Geometry check sheet. Reference: the model listing, model coordinates, mm. Face numbers are marked on the shaded views. A direction names the side the tool comes from. Round coordinates to 2 decimals unless told otherwise and drop trailing zeros. Write each loop counter-clockwise with the first axis right and the second up, starting at its lowest first coordinate (ties: lowest second). Pieces come first, ordered by that corner, then holes. Notation, with made-up numbers: M -6.75,44.5 L 38.25,44.5 A19 cw 38.25,49.5 Z; hole C -13.5,71 d4. An arc over 180 degrees is marked long. Put each result on its own line as item: value. Start each with the question number.
(1) Section check A-A on x = -205. Record the cut outline in (y, z), then the cut area to 3 significant figures.
(2) Material ranges on probe 1 along X at (y, z) = (6.5, -5); probe 2 along X at (y, z) = (47.75, -5); probe 3 along X at (y, z) = (27, -5), recorded low to high.
(3) Section check C-C on z = -5. Count the separate pieces of the cut face and the enclosed holes in it, then the cut area to 3 significant figures.
(4) Tool access check on the marked faces 1 and 2. Record the directions out of +Z, -Z, +X, -X, +Y, -Y that give a thin tool (end or side, any length) a straight path to the whole face; none if there is none.
(5) Section check D-D on x = -65. Record the cut outline in (y, z), then the cut area to 3 significant figures.
(6) Section check B-B on y = 7.5. Record the cut outline in (x, z), then the cut area to 3 significant figures.
(7) Gauge pin test, flat ends, axial feed: pin 1 (3.5 mm diameter, centred on x = 182.5, z = -5.5, fed in from -Y); pin 2 (10 mm diameter, centred on x = -139, y = 22.5, fed in from +Z); pin 3 (16 mm diameter, centred on x = 205, z = -5, fed in from +Y). Record the tip position at first contact, or that the pin passes through.
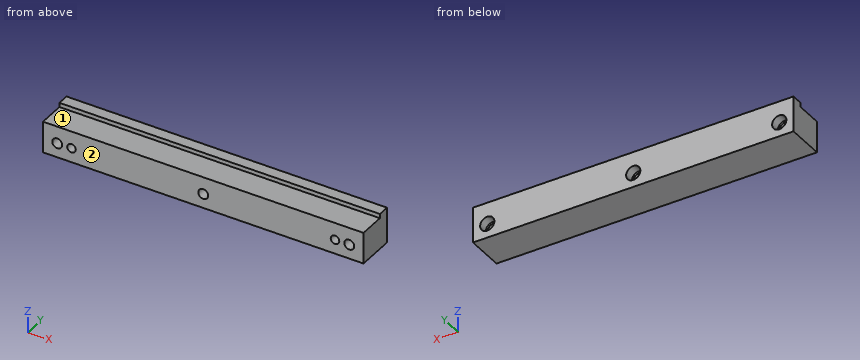
from build123d import *

# Parameters (mm, degrees)
EXTRUDE_1_DEPTH          = 225
EXTRUDE_1_DEPTH_BACK     = 225
CUT_EXTRUDE_1_DEPTH      = 233.505913903
CUT_EXTRUDE_1_DEPTH_BACK = 233.505913903
SKETCH_2_R               = 7
SKETCH_4_R               = 10
CUT_EXTRUDE_2_DEPTH      = 13
SKETCH_6_R               = 6
CUT_EXTRUDE_4_DEPTH      = 15


with BuildPart() as part:
    # Sketch 1 → Extrude 1 (new, two sides: drawn at the far end of the back side and taken through both)
    with BuildSketch(Plane(origin=(0, 0, 0), x_dir=(0, 0, -1), z_dir=(1, 0, 0)).offset(-EXTRUDE_1_DEPTH_BACK)):
        Polygon((-19, 0), (25, 0), (25, 53), (-25, 53), (-25, 37), (-19, 37), align=None)
    extrude(amount=EXTRUDE_1_DEPTH + EXTRUDE_1_DEPTH_BACK)

    # Sketch 2 → Cut-Extrude 1 (cut, two sides: drawn at the far end of the back side and taken through both)
    with BuildSketch(Plane(origin=(0, 0, 0), x_dir=(1, 0, 0), z_dir=(0, 1, 0)).offset(-CUT_EXTRUDE_1_DEPTH_BACK)):
        with Locations(Location((-205, 5, 0), (0, 0, 270))):
            Circle(SKETCH_2_R)
        with Locations(Location((0, 5, 0), (0, 0, 270))):
            Circle(SKETCH_2_R)
        with Locations(Location((205, 5, 0), (0, 0, 270))):
            Circle(SKETCH_2_R)
    extrude(amount=CUT_EXTRUDE_1_DEPTH + CUT_EXTRUDE_1_DEPTH_BACK, mode=Mode.SUBTRACT)

    # Sketch 4 → Cut-Extrude 2 (cut)
    with BuildSketch(Plane(origin=(0, 53, 0), x_dir=(1, 0, 0), z_dir=(0, 1, 0))):
        with Locations(Location((-205, 5, 0), (0, 0, 270))):
            Circle(SKETCH_4_R)
        with Locations(Location((0, 5, 0), (0, 0, 270))):
            Circle(SKETCH_4_R)
        with Locations(Location((205, 5, 0), (0, 0, 270))):
            Circle(SKETCH_4_R)
    extrude(amount=-CUT_EXTRUDE_2_DEPTH, mode=Mode.SUBTRACT)

    # Sketch 6 → Cut-Extrude 4 (cut)
    with BuildSketch(Plane(origin=(0, 0, 0), x_dir=(1, 0, 0), z_dir=(0, 1, 0))):
        with Locations(Location((-185, 5, 0), (0, 0, 270))):
            Circle(SKETCH_6_R)
        with Locations(Location((185, 5, 0), (0, 0, 270))):
            Circle(SKETCH_6_R)
    extrude(amount=CUT_EXTRUDE_4_DEPTH, mode=Mode.SUBTRACT)


solid = part.part
Answers follow:
1. outline: M 0,-25 L 53,-25 L 53,-15 L 40,-15 L 40,-12 L 0,-12 Z; M 0,2 L 40,2 L 40,5 L 53,5 L 53,25 L 37,25 L 37,19 L 0,19 Z
1. area: 1,610 mm^2
2. probe 1: x = -225 to -212, -198 to -191, -179 to -7, 7 to 179, 191 to 198, 212 to 225
2. probe 2: x = -225 to -215, -195 to -10, 10 to 195, 215 to 225
2. probe 3: x = -225 to -212, -198 to -7, 7 to 198, 212 to 225
3. separate pieces: 4
3. enclosed holes: 0
3. area: 21,000 mm^2
4. face 1: +Z, +X, -X, -Y
4. face 2: +Z, -Z, +X, -X, -Y
5. outline: M 0,-25 L 53,-25 L 53,25 L 37,25 L 37,19 L 0,19 Z
5. area: 2,430 mm^2
6. outline: M -225,-25 L 225,-25 L 225,19 L -225,19 Z; hole C -205,-5 d14; hole C -185,-5 d12; hole C 0,-5 d14; hole C 185,-5 d12; hole C 205,-5 d14
6. area: 19,100 mm^2
7. pin 1: stops at y = 15
7. pin 2: stops at z = 19
7. pin 3: stops at y = 40
